Check sheet for the modelled part. Datum: model origin and axes. Units: mm. A direction names the side the tool comes from. Round coordinates to 2 decimals unless told otherwise and drop trailing zeros. Write each loop counter-clockwise with the first axis right and the second up, starting at its lowest first coordinate (ties: lowest second). Pieces come first, ordered by that corner, then holes.
Item 1: Cross-section at B-B on x = 41.5. Enter the section's corners in (y, z), plus the area to 3 significant figures.
Item 2: Go/stop test with flat-tipped pins: pin 1 Ø5 at (x, y) = (41, -88.5) entering from -Z; pin 2 Ø3 at (y, z) = (-85.5, -7.5) entering from -X. Record where each tip stops, or that it passes through.
Item 3: Tool access check on faces 4 (the flat face through (45, -97, -6)), 5 (the flat face through (44, -94, -7)). Record the directions out of +Z, -Z, +X, -X, +Y, -Y that give a thin tool (end or side, any length) a straight path to the whole face; none if there is none.
Item 4: Release check for a two-part mould opening along Z. For faces 1 (the flat face through (52, -90, -6)), 2 (the flat face through (44, -88, 0.5)), 3 (the cylindrical face through (50.48, -84.26, -7.66)) record: +Z half, -Z half, draft (parallel to the pull), parting line (faces both ways), or undercut.
Item 5: Cross-section at D-D on x = 46. Enter the section's corners in (y, z).
Item 6: Cross-section at A-A on z = -0.25. Enter the section's corners in (x, y), plus the area to 3 significant figures.
Item 7: Cross-section at C-C on z = -7.5. Enter the section's corners in (x, y).
Item 8: Material ranges on line 1 (X direction, y = -95.8, z = -7.5); line 2 (Y direction, x = 50.1, z = -7.5); line 3 (Z direction, x = 41.5, y = -95.65), recorded low to high.
Autodesk Inventor part; units mm, degrees
ref_plane "YZ Plane" through (0, 0, 0) normal (1, 0, 0) x (0, 1, 0)
ref_plane "XZ Plane" through (0, 0, 0) normal (0, 1, 0) x (-1, 0, 0)
ref_plane "XY Plane" through (0, 0, 0) normal (0, 0, 1) x (1, 0, 0)
ref_plane "작업 평면1" through (0, 0, 0) normal (0, 0, 1) x (1, 0, 0)
sketch "스케치1" plane through (0, 0, 0) normal (0, 0, 1) x (1, 0, 0)
  line L0 (49, -94) -> (-72, -94) construction
  line L1 (49, -88) -> (49, -94) construction
  line L2 (-72, -88) -> (49, -88) construction
  line L3 (-72, -94) -> (-72, -88) construction
  line L4 (43, 88) -> (43, -88) construction
  line L5 (49, -88) -> (43, -88) construction
  line L6 (49, 88) -> (49, -88) construction
  line L7 (49, 88) -> (43, 88) construction
  line L8 (-72, -88) -> (43, -88) construction
  line L9 (43, -88) -> (43, 88) construction
  line L10 (-72, 88) -> (43, 88) construction
  line L11 (-72, 88) -> (-72, -88) construction
  circle A0 centre (-2.8299, 17.3) radius 1.35 construction
  circle A1 centre (19.1701, -17.3) radius 1.35 construction
  circle A2 centre (-24.8299, 17.3) radius 1.35 construction
  circle A3 centre (19.1701, 17.3) radius 1.35 construction
  circle A4 centre (-2.8299, -17.3) radius 1.35 construction
  circle A5 centre (-24.8299, -17.3) radius 1.35 construction
  arc A6 (-27.4299, -13.5) -> (-26.3299, -14.6) centre (-26.3299, -13.5) ccw construction
  line L12 (-27.4299, -13.5) -> (-27.4299, 13.5) construction
  arc A7 (-26.3299, 14.6) -> (-27.4299, 13.5) centre (-26.3299, 13.5) ccw construction
  line L13 (-26.3299, 14.6) -> (28.6701, 14.6) construction
  line L14 (28.6701, 14.6) -> (28.6701, -14.6) construction
  line L15 (28.6701, -14.6) -> (-26.3299, -14.6) construction
  line L16 (-72, -88) -> (43, -88) construction
  line L17 (43, -88) -> (43, 88) construction
  line L18 (-72, 88) -> (43, 88) construction
  line L19 (-72, 88) -> (-72, -88) construction
  circle A8 centre (-2.8299, 17.3) radius 1.35 construction
  circle A9 centre (19.1701, -17.3) radius 1.35 construction
  circle A10 centre (-24.8299, 17.3) radius 1.35 construction
  circle A11 centre (19.1701, 17.3) radius 1.35 construction
  circle A12 centre (-2.8299, -17.3) radius 1.35 construction
  circle A13 centre (-24.8299, -17.3) radius 1.35 construction
  arc A14 (-27.4299, -13.5) -> (-26.3299, -14.6) centre (-26.3299, -13.5) ccw construction
  line L20 (-27.4299, -13.5) -> (-27.4299, 13.5) construction
  arc A15 (-26.3299, 14.6) -> (-27.4299, 13.5) centre (-26.3299, 13.5) ccw construction
  line L21 (-26.3299, 14.6) -> (28.6701, 14.6) construction
  line L22 (28.6701, 14.6) -> (28.6701, -14.6) construction
  line L23 (28.6701, -14.6) -> (-26.3299, -14.6) construction
  line L24 (43, 88) -> (43, -88)
  line L25 (49, -88) -> (43, -88)
  line L26 (49, 88) -> (49, -88)
  line L27 (49, 88) -> (43, 88)
  line L28 (49, -94) -> (-72, -94)
  line L29 (49, -88) -> (49, -94)
  line L30 (-72, -88) -> (49, -88)
  line L31 (-72, -94) -> (-72, -88)
  line L32 (-72, -88) -> (43, -88)
  line L33 (43, -88) -> (43, 88)
  line L34 (-72, 88) -> (43, 88)
  line L35 (-72, 88) -> (-72, -88)
  circle A16 centre (-2.8299, 17.3) radius 1.35
  circle A17 centre (19.1701, -17.3) radius 1.35
  circle A18 centre (-24.8299, 17.3) radius 1.35
  circle A19 centre (19.1701, 17.3) radius 1.35
  circle A20 centre (-2.8299, -17.3) radius 1.35
  circle A21 centre (-24.8299, -17.3) radius 1.35
  arc A22 (-27.4299, -13.5) -> (-26.3299, -14.6) centre (-26.3299, -13.5) ccw
  line L36 (-27.4299, -13.5) -> (-27.4299, 13.5)
  arc A23 (-26.3299, 14.6) -> (-27.4299, 13.5) centre (-26.3299, 13.5) ccw
  line L37 (-26.3299, 14.6) -> (28.6701, 14.6)
  line L38 (28.6701, 14.6) -> (28.6701, -14.6)
  line L39 (28.6701, -14.6) -> (-26.3299, -14.6)
  line L40 (49, -94) -> (-72, -94)
  line L41 (49, -88) -> (49, -94)
  line L42 (-72, -88) -> (49, -88)
  line L43 (-72, -94) -> (-72, -88)
  line L44 (49, -94) -> (49, -77)
  line L45 (49, -94) -> (32, -94)
  line L46 (49, -77) -> (43, -77)
  line L47 (32, -94) -> (32, -88)
  line L48 (49, -94) -> (32, -94)
  line L49 (32, -94) -> (32, -77)
  line L50 (32, -77) -> (49, -77)
  line L51 (49, -77) -> (49, -94)
  line L52 (49, -94) -> (29, -94)
  line L53 (29, -94) -> (29, -77)
  line L54 (29, -77) -> (49, -77)
  line L55 (49, -77) -> (49, -94)
  point P0 (0, 0)
  dimension "d0" = 17
  dimension "d1" = 17
  dimension "d28" = 20
extrude "돌출1" add sketch "스케치1" along normal blind 3 contours L46 L26 L25 L24 | L24 L30 L49 L50 | L25 L29 L28 L47 L30 | L49 L30 L53 L54 | L47 L28 L53 L30
sketch "스케치2" plane through (49, -94, 0) normal (1, 0, 0) x (0, 0, -1)
  line L0 (40.7085, 16) -> (17.2915, 16)
  arc A0 (16.3174, 17.226) -> (17.2915, 16) centre (17.2915, 17) ccw
  line L1 (16.3174, 17.226) -> (28.0259, 67.6827)
  arc A1 (29.9741, 67.6827) -> (28.0259, 67.6827) centre (29, 67.4566) ccw
  line L2 (29.9741, 67.6827) -> (41.6826, 17.226)
  arc A2 (40.7085, 16) -> (41.6826, 17.226) centre (40.7085, 17) ccw
  line L3 (34.1853, 94.226) -> (45.1259, 141.3733)
  arc A3 (47.1, 141.1472) -> (45.1259, 141.3733) centre (46.1, 141.1472) ccw
  line L4 (47.1, 141.1472) -> (47.1, 46.8528)
  arc A4 (45.1259, 46.6267) -> (47.1, 46.8528) centre (46.1, 46.8528) ccw
  line L5 (45.1259, 46.6267) -> (34.1853, 93.774)
  arc A5 (34.1853, 94.226) -> (34.1853, 93.774) centre (35.1594, 94) ccw
  line L6 (10.9, 46.8528) -> (10.9, 141.1472)
  arc A6 (12.8741, 141.3733) -> (10.9, 141.1472) centre (11.9, 141.1472) ccw
  line L7 (12.8741, 141.3733) -> (23.8147, 94.226)
  arc A7 (23.8147, 93.774) -> (23.8147, 94.226) centre (22.8406, 94) ccw
  line L8 (23.8147, 93.774) -> (12.8741, 46.6267)
  arc A8 (10.9, 46.8528) -> (12.8741, 46.6267) centre (11.9, 46.8528) ccw
  line L9 (28.0259, 120.3173) -> (16.3174, 170.774)
  arc A9 (17.2915, 172) -> (16.3174, 170.774) centre (17.2915, 171) ccw
  line L10 (17.2915, 172) -> (40.7085, 172)
  arc A10 (41.6826, 170.774) -> (40.7085, 172) centre (40.7085, 171) ccw
  line L11 (41.6826, 170.774) -> (29.9741, 120.3173)
  arc A11 (28.0259, 120.3173) -> (29.9741, 120.3173) centre (29, 120.5434) ccw
  line L12 (58, 182) -> (0, 182)
  line L13 (0, 182) -> (0, 6)
  line L14 (58, 6) -> (0, 6)
  line L15 (58, 6) -> (58, 182)
  line L16 (58, 0) -> (0, 0)
  line L17 (58, 6) -> (58, 0)
  line L18 (0, 6) -> (58, 6)
  line L19 (0, 6) -> (0, 0)
  line L20 (6, 182) -> (6, 6)
  line L21 (0, 0) -> (0, 17)
  line L22 (0, 17) -> (-3, 17)
  line L23 (-3, 0) -> (-3, 17)
  line L24 (0, 0) -> (-3, 0)
  line L25 (-3, 0) -> (22, 0)
  line L26 (22, 0) -> (22, 17)
  line L27 (22, 17) -> (-3, 17)
  line L28 (-3, 17) -> (-3, 0)
  point P0 (0, 94)
  point P1 (0, 0)
  point P2 (22, 0)
  point P3 (22, 16)
  point P4 (16.2915, 17)
  point P5 (0, 17)
  dimension "d4" = 25
extrude "돌출2" add sketch "스케치2" along normal blind 3 contours L26 L14 L20 L27 A0 L0 | L0 A0 L27 L26 | L26 L16 L19 L14 | L14 L13 L27 L20 | L19 L24 L23 L22 L13
sketch "스케치3" plane through (32, -94, 0) normal (0, -1, 0) x (1, 0, 0)
  line L0 (20, 3) -> (20, -22)
  line L1 (0, 0) -> (0, 3)
  line L2 (20, -22) -> (0, -22)
  line L3 (0, -22) -> (0, 3)
  line L4 (0, 3) -> (20, 3)
  line L5 (20, 3) -> (20, -22)
  line L6 (20, 3) -> (-3, 3)
  line L7 (-3, 3) -> (-3, -22)
  line L8 (-3, -22) -> (20, -22)
  line L9 (20, -22) -> (20, 3)
  point P0 (-32, 0)
  point P1 (20, 3)
  point P2 (0, -22)
  dimension "d27" = 23
extrude "돌출3" add sketch "스케치3" along normal blind 3
sketch "스케치8" plane through (0, 0, 3) normal (0, 0, 1) x (1, 0, 0)
  line L0 (29, -97) -> (52, -97)
  line L1 (29, -77) -> (52, -77)
  line L2 (52, -97) -> (34, -97)
  line L3 (34, -97) -> (34, -77)
  line L4 (34, -77) -> (52, -77)
  line L5 (52, -77) -> (52, -97)
  line L6 (34, -77) -> (29, -77)
  line L7 (29, -77) -> (29, -97)
  line L8 (29, -97) -> (34, -97)
  line L9 (34, -97) -> (34, -77)
  point P0 (0, 0)
  dimension "d29" = 18
extrude "돌출8" cut sketch "스케치8" against normal blind 50 contours L7 L1 L3 L0
sketch "스케치10" plane through (52, -94, 0) normal (1, 0, 0) x (0, 0, -1)
  line L0 (-3, 17) -> (-3, -3)
  line L1 (22, -3) -> (-3, -3)
  line L2 (-3, 17) -> (17, 17)
  line L3 (17, 17) -> (17, -3)
  line L4 (17, -3) -> (-3, -3)
  line L5 (-3, -3) -> (-3, 17)
  line L6 (-3, 17) -> (15, 17)
  line L7 (15, 17) -> (15, -3)
  line L8 (15, -3) -> (-3, -3)
  line L9 (-3, -3) -> (-3, 17)
  line L10 (15, 17) -> (22, 17)
  line L11 (22, 17) -> (22, -3)
  line L12 (22, -3) -> (15, -3)
  line L13 (15, -3) -> (15, 17)
  point P0 (0, 94)
  point P1 (15, 17)
  point P2 (17, 17)
  dimension "d32" = 20
  dimension "d33" = 18
extrude "돌출9" cut sketch "스케치10" against normal blind 50 contours L2 L3 L1 L7 | L10 L11 L1 L3
sketch "스케치12" plane through (32, -94, 0) normal (0, 1, 0) x (1, 0, 0)
  circle A0 centre (14, 1) radius 1.25
  circle A1 centre (8, 17) radius 1.25
  circle A2 centre (8, 1) radius 1.25
  circle A3 centre (14, 17) radius 1.25
  line L0 (4, -3) -> (20, -3)
  line L1 (20, 21) -> (20, -3)
  line L2 (4, 21) -> (20, 21)
  line L3 (4, 21) -> (4, -3)
  circle A4 centre (14, 1) radius 1.25
  arc A5 (8.2846, 1.2694) -> (7.5179, 0.8668) centre (7.785, 1.2894) ccw
  point P0 (-32, 0)
extrude "돌출10" cut sketch "스케치12" against normal blind 50 contours A0
sketch "스케치13" plane through (0, 0, 0) normal (0, 0, -1) x (-1, 0, 0)
  line L0 (-34, -94) -> (-34, -77)
  line L1 (-49, -77) -> (-34, -77)
  line L2 (-49, -94) -> (-49, -77)
  line L3 (-46.75, -94) -> (-49, -94)
  line L4 (-45.25, -94) -> (-46.75, -94)
  line L5 (-34, -94) -> (-45.25, -94)
  line L6 (-41.5, -94) -> (-41.5, -77)
  line L7 (-34, -85.5) -> (-49, -85.5)
  circle A0 centre (-41.5, -85.5) radius 1.25
  point P0 (0, 0)
  dimension "d38" = 2.5
extrude "돌출11" cut sketch "스케치13" against normal blind 50 contours A0 L6 L7 | L7 L6 A0 | A0 L7 L6 | L7 A0 L6
sketch "스케치14" plane through (49, -94, 0) normal (-1, 0, 0) x (0, 0, 1)
  line L0 (-15, 17) -> (-15, 0)
  line L1 (0, 0) -> (-15, 0)
  line L2 (0, 0) -> (0, 17)
  line L3 (-15, 17) -> (0, 17)
  line L4 (-15, 8.5) -> (0, 8.5)
  line L5 (0, 0) -> (-15, 0)
  line L6 (-7.5, 0) -> (-7.5, 17)
  circle A0 centre (-7.5, 8.5) radius 1.25
  point P0 (0, 94)
  dimension "d41" = 2.5
extrude "돌출12" cut sketch "스케치14" against normal blind 50 contours A0 L6 L4 | L4 L6 A0 | A0 L4 L6 | L4 A0 L6
sketch "스케치15" plane through (32, -94, 0) normal (0, 1, 0) x (1, 0, 0)
  line L0 (2, 0) -> (13.25, 0)
  arc A0 (14.75, 0) -> (13.25, 0) centre (14, 1) ccw
  line L1 (14.75, 0) -> (17, 0)
  line L2 (17, 0) -> (17, 15)
  line L3 (17, 15) -> (2, 15)
  line L4 (2, 15) -> (2, 0)
  line L5 (9.5, 15) -> (9.5, 0)
  line L6 (8.75, 0) -> (13.25, 0)
  line L7 (2, 15) -> (2, 0)
  line L8 (2, 7.5) -> (17, 7.5)
  circle A1 centre (9.5, 7.5) radius 1.25
  point P0 (-32, 0)
  dimension "d44" = 2.5
extrude "돌출13" cut sketch "스케치15" against normal blind 50 contours A1 L5 L8 | L8 L5 A1 | L5 L8 A1 | L5 A1 L8
sketch "스케치16" plane through (0, 0, 0) normal (0, 0, -1) x (-1, 0, 0)
  circle A0 centre (-41.5, -85.5) radius 1.25
  line L0 (-34, -94) -> (-34, -77)
  line L1 (-49, -77) -> (-34, -77)
  line L2 (-49, -94) -> (-49, -77)
  line L3 (-46.75, -94) -> (-49, -94)
  line L4 (-45.25, -94) -> (-46.75, -94)
  line L5 (-34, -94) -> (-45.25, -94)
  point P0 (0, 0)
extrude "돌출14" cut sketch "스케치16" against normal blind 0.5
sketch "스케치17" plane through (52, -97, -15) normal (0, 0, -1) x (-1, 0, 0)
  line L0 (18, 20) -> (18, 0)
  line L1 (0, 0) -> (18, 0)
  line L2 (18, 20) -> (13.0164, 20)
  line L3 (13.0164, 20) -> (13.0164, 0)
  line L4 (13.0164, 0) -> (18, 0)
  line L5 (18, 0) -> (18, 20)
  point P0 (52, 97)
extrude "돌출15" cut sketch "스케치17" against normal blind 50
sketch "스케치18" plane through (52, -97, -15) normal (0, 0, -1) x (-1, 0, 0)
  line L0 (0, 20) -> (0, 0)
  line L1 (13.0164, 20) -> (13.0164, 0)
  line L2 (0, 20) -> (13.0164, 20)
  line L3 (13.0164, 20) -> (13.0164, 14.3347)
  line L4 (13.0164, 14.3347) -> (0, 14.3347)
  line L5 (0, 14.3347) -> (0, 20)
  point P0 (52, 97)
extrude "돌출16" cut sketch "스케치18" against normal blind 50
properties part number "body_fitting_part_under" material "LCP 플라스틱"
Response values:
1. outline: (-97, -15) - (-94, -15) - (-94, -8.75) - (-97, -8.75) - close; (-97, -6.25) - (-94, -6.25) - (-94, 0.5) - (-86.75, 0.5) - (-86.75, 3) - (-97, 3) - close; (-84.25, 0.5) - (-82.67, 0.5) - (-82.67, 3) - (-84.25, 3) - close
1. area: 68.6 mm2
2. pin 1: stops at z = 0.5
2. pin 2: stops at x = 49
3. face 4: +Z, -Z, +X, -X, -Y
3. face 5: -Z, -X, +Y
4. face 1: draft
4. face 2: -Z half
4. face 3: undercut
5. outline: (-97, -15) - (-94, -15) - (-94, -2.25) - (-97, -2.25) - close; (-97, 0.25) - (-94, 0.25) - (-94, 0.5) - (-82.67, 0.5) - (-82.67, 3) - (-97, 3) - close
6. outline: (38.98, -97) - (45, -97) - (45, -94) - (38.98, -94) - close; (47, -97) - (52, -97) - (52, -82.67) - (49, -82.67) - (49, -94) - (47, -94) - close
6. area: 67.1 mm2
7. outline: (38.98, -97) - (40.25, -97) - (40.25, -94) - (38.98, -94) - close; (42.75, -97) - (52, -97) - (52, -86.75) - (49, -86.75) - (49, -94) - (42.75, -94) - close; (49, -84.25) - (52, -84.25) - (52, -82.67) - (49, -82.67) - close
8. line 1: x = 38.98 to 40.25, 42.75 to 52
8. line 2: y = -97 to -86.75, -84.25 to -82.67
8. line 3: z = -15 to -8.75, -6.25 to 3
